Part model, mm, in its own coordinate system. Face numbers are marked on the shaded views. A direction names the side the tool comes from. Coordinates: 2 decimals unless noted, no trailing zeros. Order: outer loops, then holes, each group sorted by start corner. A loop starts at its lowest first (then second) coordinate and runs counter-clockwise, first axis right, second up.
1) Tool access for the marked faces 1, 2, 3 and 4: list every direction of +Z, -Z, +X, -X, +Y, -Y with a clear straight run to the whole face (end or side of a thin tool).
2) Cut at A-A (z = 12). List the corners of the cut face in (x, y).
3) Pin check, flat tips, straight feed: pin 1 Ø1 at (x, y) = (-44.5, 28.5) entering from -Z; pin 2 Ø1.1 at (x, y) = (10, -28) entering from -Z; pin 3 Ø8 at (x, z) = (43.5, 12) entering from -Y; pin 4 Ø0.5 at (x, y) = (-40.5, -4) entering from -Z. Stop position of each tip, or through.
4) Cut at D-D (y = 19). List the corners of the cut face in (x, z).
5) Cut at C-C (y = 4). List the corners of the cut face in (x, z), and give its area (3 significant figures).
6) Wall check: L1, parallel to X at y = 26, z = 19.25; L2, parallel to Y at x = -37, z = 6; L3, parallel to X at y = -9, z = 3.5. Give the ranges that are in metal, low to high.
7) Cut at B-B (x = -16). List the corners of the cut face in (y, z), and give its area (3 significant figures).
```python
from build123d import *

# Parameters (mm, degrees)
SKETCH_1_W          = 80
SKETCH_1_H          = 55
EXTRUDE_1_DEPTH     = 20
EXTRUDE_2_DEPTH     = 2
SKETCH_3_W          = 95
SKETCH_3_H          = 2
EXTRUDE_3_DEPTH     = 55
EXTRUDE_4_DEPTH     = 30
CUT_EXTRUDE_1_DEPTH = 84.458073306
CUT_EXTRUDE_2_DEPTH = 65.058566952
FILLET_1_R          = 3
EXTRUDE_5_DEPTH     = 15


with BuildPart() as part:
    # Sketch 1 → Extrude 1 (new body)
    with BuildSketch(Plane.XY):
        Rectangle(SKETCH_1_W, SKETCH_1_H)
    extrude(amount=EXTRUDE_1_DEPTH)



with BuildPart() as body_2:
    # Sketch 2 → Extrude 2 (new body)
    with BuildSketch(Plane(origin=(0, 27.5, 0), x_dir=(1, 0, 0), z_dir=(0, 1, 0))):
        Polygon((-47.5, 0), (-47.5, -22), (47.5, -22), (47.5, 0), (40, 0), (-40, 0), align=None)
    extrude(amount=EXTRUDE_2_DEPTH)


with BuildPart() as part_1:
    add(part.part)

    add(body_2.part)  # Extrude 3 merges body 2
    # Sketch 3 → Extrude 3 (add)
    with BuildSketch(Plane.XZ.offset(-27.5)):
        with Locations((0, 21)):
            Rectangle(SKETCH_3_W, SKETCH_3_H)
    extrude(amount=EXTRUDE_3_DEPTH)

    # Sketch 4 → Extrude 4 (add, symmetric)
    with BuildSketch(Plane(origin=(0, 0, 0), x_dir=(0, 0, -1), z_dir=(1, 0, 0))):
        Polygon((-1, -27.5), (-1, -28.5), (1, -28.5), (1, -37.5), (-14, -37.5), (-14, -27.5), align=None)
    extrude(amount=EXTRUDE_4_DEPTH, both=True)

    # Sketch 5 → Cut-Extrude 1 (cut, through all)
    with BuildSketch(Plane.XZ.offset(-27.5)):
        with BuildLine():
            Line((52.5, 10), (42.5, 10))
            ThreePointArc((42.5, 10), (40.5, 12), (42.5, 14))
            Line((42.5, 14), (52.5, 14))
            ThreePointArc((52.5, 14), (54.5, 12), (52.5, 10))
        make_face()
    cut_extrude_1 = extrude(amount=-CUT_EXTRUDE_1_DEPTH, mode=Mode.SUBTRACT)

    # Sketch 6 → Cut-Extrude 2 (cut, through all)
    with BuildSketch(Plane(origin=(0, 0, 20), x_dir=(-1, 0, 0), z_dir=(0, 0, -1))):
        with BuildLine():
            Line((-52.5, 2.5), (-42.5, 2.5))
            ThreePointArc((-42.5, 2.5), (-40.5, 0.5), (-42.5, -1.5))
            Line((-42.5, -1.5), (-52.5, -1.5))
            ThreePointArc((-52.5, -1.5), (-54.5, 0.5), (-52.5, 2.5))
        make_face()
    cut_extrude_2 = extrude(amount=-CUT_EXTRUDE_2_DEPTH, mode=Mode.SUBTRACT)

    # Mirror 1: Cut-Extrude 1, Cut-Extrude 2 across plane
    add(cut_extrude_1.mirror(Plane(origin=(0, 0, 0), x_dir=(0, 0, 1), z_dir=(1, 0, 0))), mode=Mode.SUBTRACT)
    add(cut_extrude_2.mirror(Plane(origin=(0, 0, 0), x_dir=(0, 0, 1), z_dir=(1, 0, 0))), mode=Mode.SUBTRACT)

    # Fillet 1
    fillet_1_edges = [part_1.edges().sort_by_distance(p)[0] for p in [
        (47.5, -27.5, 21),
        (-47.5, -27.5, 21),
        (47.5, 28.5, 0),
        (-47.5, 28.5, 0),
    ]]
    fillet(fillet_1_edges, radius=FILLET_1_R)

    # Sketch 7 → Extrude 5 (add)
    with BuildSketch(Plane(origin=(0, 5.5, 0), x_dir=(-1, 0, 0), z_dir=(0, -1, 0))):
        Polygon((40, -1), (41, -1), (41, 1), (50, 1), (50, -14), (40, -14), align=None)
    extrude(amount=EXTRUDE_5_DEPTH)


solid = part_1.part
```
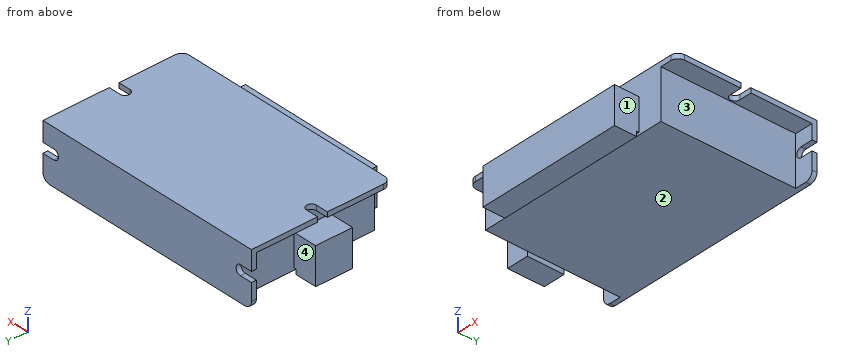
Geometry check:
1. face 1: +Z, -Z, +X, -Y
1. face 2: -Z, +X, +Y
1. face 3: -Z, +X, -Y
1. face 4: -Z, -X
2. outline: (-50, -9.5) - (-40, -9.5) - (-40, -27.5) - (-30, -27.5) - (-30, -37.5) - (30, -37.5) - (30, -27.5) - (40, -27.5) - (40, 27.5) - (40.5, 27.5) - (40.5, 29.5) - (-40.5, 29.5) - (-40.5, 27.5) - (-40, 27.5) - (-40, 5.5) - (-50, 5.5) - close
3. pin 1: stops at z = 0
3. pin 2: stops at z = -1
3. pin 3: stops at y = -27.5
3. pin 4: stops at z = 1
4. outline: (-47.5, 20) - (-40, 20) - (-40, 0) - (40, 0) - (40, 20) - (47.5, 20) - (47.5, 22) - (-47.5, 22) - close
5. outline: (-50, -1) - (-41, -1) - (-41, 1) - (-40, 1) - (-40, 0) - (40, 0) - (40, 20) - (47.5, 20) - (47.5, 22) - (-47.5, 22) - (-47.5, 20) - (-40, 20) - (-40, 14) - (-50, 14) - close
5. area: 1,940 mm2
6. L1: x = -40 to 40
6. L2: y = -27.5 to 29.5
6. L3: x = -50 to 40
7. outline: (-37.5, -1) - (-28.5, -1) - (-28.5, 1) - (-27.5, 1) - (-27.5, 0) - (29.5, 0) - (29.5, 22) - (-27.5, 22) - (-27.5, 14) - (-37.5, 14) - close
7. area: 1,400 mm2
